Read the model definition and answer for the solid it produces. Units are mm, in the model's axes. A direction names the side the tool comes from. Coordinates: 2 decimals unless noted, no trailing zeros. Loops run counter-clockwise (first coordinate to the right, second up) from the corner with the lowest first, then second, coordinate; pieces in that order, holes last. Notation, with made-up numbers: (34.25, 86.5) - (38.25, 86.5) arc R26 cw to (38.25, 125.5) - close; hole circle Ø3 at (87, 80). An arc over 180 degrees is marked (long way). One line per item, written item: value. Start each with the question number.
from build123d import *

# Parameters (mm, degrees)
BOSS_EXTRUDE3_DEPTH   = 15.38
BOSS_EXTRUDE3_2_DEPTH = 15.38
BOSS_EXTRUDE3_3_DEPTH = 15.38
BOSS_EXTRUDE5_DEPTH   = 3


with BuildPart() as part:
    # Sketch1 → Boss-Extrude3 (new body)
    with BuildSketch(Plane(origin=(0, 0, 0), x_dir=(1, 0, 0), z_dir=(0, 1, 0))):
        Polygon((-130.752776749, -1.17820323), (-148.526279441, -1.17820323), (-138.959292143, 15.392304845), (-130.072540797, 0), align=None)
        Polygon((-144.196152422, 1.32179677), (-138.959292143, 10.392304845), (-133.722431864, 1.32179677), align=None, mode=Mode.SUBTRACT)
    extrude(amount=BOSS_EXTRUDE3_DEPTH)



with BuildPart() as body_2:
    # Sketch1 → Boss-Extrude3 2 (new body)
    with BuildSketch(Plane(origin=(0, 0, 0), x_dir=(1, 0, 0), z_dir=(0, 1, 0))):
        Polygon((-138.959292143, -29.498711305), (-130.072540797, -14.106406459), (-130.752776749, -12.92820323), (-148.526279441, -12.92820323), align=None)
        Polygon((-144.196152422, -15.42820323), (-133.722431864, -15.42820323), (-138.959292143, -24.498711305), align=None, mode=Mode.SUBTRACT)
    extrude(amount=BOSS_EXTRUDE3_2_DEPTH)


with BuildPart() as body_3:
    # Sketch1 → Boss-Extrude3 3 (new body)
    with BuildSketch(Plane(origin=(0, 0, 0), x_dir=(1, 0, 0), z_dir=(0, 1, 0))):
        Polygon((-118.536270399, -19.981406459), (-109.649519053, -35.373711305), (-128.783493648, -35.373711305), (-119.896742302, -19.981406459), align=None)
        Polygon((-113.979646072, -32.873711305), (-124.453366629, -32.873711305), (-119.216506351, -23.80320323), align=None, mode=Mode.SUBTRACT)
    extrude(amount=BOSS_EXTRUDE3_3_DEPTH)


with BuildPart() as part_1:
    add(part.part)

    add(body_2.part)  # Boss-Extrude5 merges body 2

    add(body_3.part)  # Boss-Extrude5 merges body 3
    # Sketch1_7 → Boss-Extrude5 (add)
    with BuildSketch(Plane(origin=(0, 0, 0), x_dir=(1, 0, 0), z_dir=(0, 1, 0))):
        Polygon((-118.536270399, -19.981406459), (-130.072540797, 0), (-130.752776749, -1.17820323), (-148.526279441, -1.17820323), (-139.639528095, -7.05320323), (-148.526279441, -12.92820323), (-130.752776749, -12.92820323), (-130.072540797, -14.106406459), (-138.959292143, -29.498711305), (-129.428017223, -24.740058882), (-128.783493648, -35.373711305), (-119.896742302, -19.981406459), align=None)
    extrude(amount=BOSS_EXTRUDE5_DEPTH)


solid = part_1.part
1) Section D-D, the plane y = 1.75 is taken. Determine the outline of the cut face in (x, z), and give its area (3 significant figures).
2) Section C-C, the plane x = -142.5 is taken. Determine the outline of the cut face in (y, z).
3) Section B-B, the plane z = 21 is taken. Determine the outline of the cut face in (x, y), and give its area (3 significant figures).
4) Section A-A, the plane y = 12.25 is taken. Determine the outline of the cut face in (x, z).
5) Flat-ended cylindrical pins translate along their axes: P1, Ø3, axis at x = -117, y = 9.5, coming from the -Z side; P2, Ø1, axis at y = 1.5, z = 11, coming from the -X side; P3, Ø2, axis at x = -122, z = 14, coming from the +Y side. Find the tip coordinate at first contact, or state that the pin passes through.
6) Determine the mould class of faces 4 (the flat face through (-144.02, 1.48, 9.95)), 5 (the flat face through (-119, 9, 19.981)), 6 (the flat face through (-116.635, 7.582, 28.275)) for opening direction X: released by +X, released by -X, zero draft, split by the parting line, or undercut.
7) Straight lines are drawn through the part: L1, parallel to Z at x = -136, y = 11; L2, parallel to X at y = 13.25, z = 28; L3, parallel to Z at x = -131, y = 4.5. For each, find the intervals that lie inside material, in ascending order.
8) For faces 1 (the flat face through (-140, 9, 1.178)), 2 (the flat face through (-134.58, 9.1, 21.91)), 3 (the flat face through (-139, 8, -1.322)), determine the directions among +Z, -Z, +X, -X, +Y, -Y from which every point of the face is accessible in a straight line to the end or side of a thin tool.
Answer below:
1. outline: (-148.53, 1.18) - (-138.96, -15.39) - (-109.65, 35.37) - (-128.78, 35.37) - (-129.43, 24.74) - (-138.96, 29.5) - (-148.53, 12.93) - (-139.64, 7.05) - close; hole (-144.2, -1.32) - (-138.96, -10.39) - (-133.72, -1.32) - close; hole (-144.2, 15.43) - (-133.72, 15.43) - (-138.96, 24.5) - close; hole (-124.45, 32.87) - (-119.22, 23.8) - (-113.98, 32.87) - close
1. area: 738 mm2
2. outline: (0, -9.26) - (15.38, -9.26) - (15.38, -4.26) - (0, -4.26) - close; (0, -1.32) - (15.38, -1.32) - (15.38, 1.18) - (3, 1.18) - (3, 5.16) - (0, 5.16) - close; (0, 8.94) - (3, 8.94) - (3, 12.93) - (15.38, 12.93) - (15.38, 15.43) - (0, 15.43) - close; (0, 18.37) - (15.38, 18.37) - (15.38, 23.37) - (0, 23.37) - close
3. outline: (-143.87, 0) - (-140.98, 0) - (-140.98, 15.38) - (-143.87, 15.38) - close; (-136.94, 0) - (-117.95, 0) - (-117.95, 15.38) - (-120.48, 15.38) - (-120.48, 3) - (-134.05, 3) - (-134.05, 15.38) - (-136.94, 15.38) - close
3. area: 169 mm2
4. outline: (-148.53, 1.18) - (-138.96, -15.39) - (-130.07, 0) - (-130.75, 1.18) - close; (-148.53, 12.93) - (-130.75, 12.93) - (-130.07, 14.11) - (-138.96, 29.5) - close; (-128.78, 35.37) - (-119.9, 19.98) - (-118.54, 19.98) - (-109.65, 35.37) - close; hole (-144.2, -1.32) - (-138.96, -10.39) - (-133.72, -1.32) - close; hole (-144.2, 15.43) - (-133.72, 15.43) - (-138.96, 24.5) - close; hole (-124.45, 32.87) - (-119.22, 23.8) - (-113.98, 32.87) - close
5. P1: z = 20.04
5. P2: x = -146.37
5. P3: y = 3
6. face 4: released by -X
6. face 5: zero draft
6. face 6: undercut
7. L1: -10.27 to -5.27, -1.32 to 1.18, 12.93 to 15.43, 19.37 to 24.37
7. L2: -139.82 to -138.09, -124.53 to -121.64, -116.79 to -113.91
7. L3: -1.61 to 1.18, 12.93 to 15.71
8. face 1: +X, -X, +Y
8. face 2: +Z, +Y
8. face 3: +Y, -Y
